Geometry check sheet. Reference: the model listing, model coordinates, mm. A direction names the side the tool comes from. Give positions to 0.01 mm unless a question says otherwise; leave off trailing zeros.
from build123d import *

# Parameters (mm, degrees)
SHELL1_T               = -2
BOSS_EXTRUDE1_START    = 2
SKETCH7_4_W            = 2
SKETCH7_4_H            = 2.3
BOSS_EXTRUDE1_DEPTH    = 50.7
FILLET1_R              = 2.4
CUT_EXTRUDE1_START     = -40.445352697
CUT_EXTRUDE1_OUTLINE_W = 62.3
CUT_EXTRUDE1_OUTLINE_H = 22.2
CUT_EXTRUDE1_DEPTH     = 6.532429258
BOSS_EXTRUDE2_DEPTH    = 1
SKETCH11_R             = 2.25
CUT_EXTRUDE2_DEPTH     = 2
SKETCH12_R             = 1.875
CUT_EXTRUDE3_DEPTH     = 2


# Read off the part's stored shape, not the designer's step: Cut-Extrude1
with BuildPart() as part:
    # Sketch7 → Loft1 section 0
    with BuildSketch(Plane(origin=(0, 0, 0), x_dir=(1, 0, 0), z_dir=(0, 1, 0))):
        with BuildLine():
            Line((0, 66.4), (32.183064352, 66.4))
            ThreePointArc((32.183064352, 66.4), (36.140979043, 33.2), (32.183064352, 0))
            Line((32.183064352, 0), (0, 0))
            Line((0, 0), (0, 66.4))
        make_face()
    # Sketch1 → Loft1 section 1
    with BuildSketch(Plane(origin=(0, 93, 0), x_dir=(1, 0, 0), z_dir=(0, 1, 0))):
        with BuildLine():
            Line((0, 66.4), (0, 0))
            Line((0, 0), (36.793809788, 0))
            ThreePointArc((36.793809788, 0), (40.63882203, 33.2), (36.793809788, 66.4))
            Line((36.793809788, 66.4), (0, 66.4))
        make_face()
    loft()

    # Shell1
    shell1_openings = [part.faces().sort_by_distance(p)[0] for p in [
        (19.698634873, 93, -33.2),
    ]]
    offset(amount=SHELL1_T, openings=shell1_openings, kind=Kind.INTERSECTION)

    # Sketch7<4> → Boss-Extrude1 (add)
    with BuildSketch(Plane(origin=(0, 0, 0), x_dir=(1, 0, 0), z_dir=(0, 1, 0)).offset(BOSS_EXTRUDE1_START)):
        Polygon((2, 35.2), (2, 33.2), (24.2, 33.2), (24.2, 2), (26.2, 2), (26.2, 35.2), (5.4, 35.2), (3.4, 35.2), align=None)
        with Locations((4.4, 36.35)):
            Rectangle(SKETCH7_4_W, SKETCH7_4_H)
        with Locations((4.4, 63.25)):
            Rectangle(SKETCH7_4_W, SKETCH7_4_H)
    extrude(amount=BOSS_EXTRUDE1_DEPTH)

    # Fillet1
    # the kernel refuses this fillet: 2.4 mm, written as the material it adds along each edge
    with BuildSketch(Plane(origin=(5.4, 2, -35.2), x_dir=(1, 0, 0), z_dir=(0, 1, 0))) as fillet1_piece_1:
        with BuildLine():
            CenterArc((2.397915762, 2.4), FILLET1_R, 182.388015463, 87.611984537)
            Line((0, 2.3), (-0.047958315, 2.298))
            ThreePointArc((-0.047958315, 2.298), (-0.048, 1.15), (-0.048, 0))
            Line((-0.048, 0), (0, -0.048))
            Line((0, -0.048), (2.397915762, -0.048))
            Line((2.397915762, -0.048), (2.397915762, 0))
        make_face()
    extrude(amount=50.7)
    with BuildSketch(Plane(origin=(5.4, 2, -64.4), x_dir=(1, 0, 0), z_dir=(0, 1, 0))) as fillet1_piece_2:
        with BuildLine():
            CenterArc((2.397915762, -2.4), FILLET1_R, 90, 87.611984537)
            Line((0, -2.3), (-0.047958315, -2.298))
            ThreePointArc((-0.047958315, -2.298), (-0.048, -1.15), (-0.048, 0))
            Line((-0.048, 0), (0, 0.048))
            Line((0, 0.048), (2.397915762, 0.048))
            Line((2.397915762, 0.048), (2.397915762, 0))
        make_face()
    extrude(amount=50.7)

    # Cut-Extrude1 outline → Cut-Extrude1 (cut)
    with BuildSketch(Plane.ZY.offset(CUT_EXTRUDE1_START)):
        with Locations((-33.2, 77.9)):
            Rectangle(CUT_EXTRUDE1_OUTLINE_W, CUT_EXTRUDE1_OUTLINE_H)
    extrude(amount=CUT_EXTRUDE1_DEPTH, mode=Mode.SUBTRACT)

    # Sketch10 → Boss-Extrude2 (add, symmetric)
    with BuildSketch(Plane(origin=(17, 0, 0), x_dir=(0, 0, -1), z_dir=(1, 0, 0))):
        Polygon((62.578627716, 89), (64.578627716, 83.505045161), (64.578627716, 89), align=None)
    boss_extrude2 = extrude(amount=BOSS_EXTRUDE2_DEPTH, both=True)

    # Sketch11 → Cut-Extrude2 (cut)
    with BuildSketch(Plane(origin=(0, 0, -66.4), x_dir=(-1, 0, 0), z_dir=(0, 0, -1))):
        with Locations((-16.091532176, 50.25)):
            Circle(SKETCH11_R)
    extrude(amount=-CUT_EXTRUDE2_DEPTH, mode=Mode.SUBTRACT)

    # Sketch12 → Cut-Extrude3 (cut)
    with BuildSketch(Plane(origin=(0, 0, -2), x_dir=(-1, 0, 0), z_dir=(0, 0, -1))):
        with Locations((-29.702128484, 52.7)):
            Circle(SKETCH12_R)
    extrude(amount=-CUT_EXTRUDE3_DEPTH, mode=Mode.SUBTRACT)

    # Mirror1: Boss-Extrude2 across plane
    add(boss_extrude2.mirror(Plane.XY.offset(-33.2)))


solid = part.part
Item 1: Draft check along Z on faces 1 (the flat face through (16, 0, -33)), 2 (the flat face through (3.4, 27, -63)). Enter one of: released by +Z, released by -Z, zero draft, split by the parting line, or undercut.
Reported:
face 1: zero draft
face 2: undercut
Item 2: Set-up check for faces 3 (the flat face through (17, 89, -3)), 4 (the cylindrical face through (14.882, 52.147, -65.414)), 5 (the flat face through (38, 66.8, -34)): record each of +Z, -Z, +X, -X, +Y, -Y from which the full face is reachable in a straight line by a thin tool's end or side.
Reported:
face 3: +Y
face 4: -Z
face 5: +X
Item 3: Scan lines: L1, parallel to X at y = 11, z = -7; L2, parallel to Z at x = 14, y = 33; L3, parallel to Z at x = 32, y = 50. Record each from-to range of solid material in increasing order.
Reported:
L1: x = 0 to 2, 24.2 to 26.2, 32.19 to 34.23
L2: z = -66.4 to -64.4, -35.2 to -33.2, -2 to 0
L3: z = -66.4 to -64.4, -2 to 0
Item 4: Gauge pin test, flat ends, axial feed: pin 1 (2 mm diameter, centred on y = 85.5, z = -64, fed in from +X); pin 2 (6.5 mm diameter, centred on x = 10, z = -22, fed in from +Y); pin 3 (0.5 mm diameter, centred on x = 16.5, z = -3, fed in from +Y). Record the tip position at first contact, or that the pin passes through.
Reported:
pin 1: stops at x = 36.94
pin 2: stops at y = 2
pin 3: stops at y = 89
Item 5: Sectioned sample at A-A (y = 38). Give the number of separate pieces and of enclosed holes in the cut face, and give its area (3 significant figures).
Reported:
separate pieces: 1
enclosed holes: 2
area: 510 mm2
